```python
from build123d import *

# Parameters (mm, degrees)
SKETCH2_R           = 3.2639
BOSS_EXTRUDE1_DEPTH = 25.0031
SKETCH3_R           = 15.875
CUT_EXTRUDE1_DEPTH  = 13.7
CHAMFER1_SIZE       = 0.5
CHAMFER2_SIZE       = 0.5


with BuildPart() as part:
    # Sketch2 → Boss-Extrude1 (new body)
    with BuildSketch(Plane.XY):
        with BuildLine():
            Line((-6.35, 23.8125), (-6.35, -23.8114))
            ThreePointArc((-6.35, -23.8114), (0, -30.1614), (6.35, -23.8114))
            Line((6.35, -23.8114), (6.35, 23.8125))
            ThreePointArc((6.35, 23.8125), (0, 30.1625), (-6.35, 23.8125))
        make_face()
        with Locations((0, -23.8114)):
            Circle(SKETCH2_R, mode=Mode.SUBTRACT)
        with Locations((0, 23.8125)):
            Circle(SKETCH2_R, mode=Mode.SUBTRACT)
    extrude(amount=BOSS_EXTRUDE1_DEPTH)

    # Sketch3 → Cut-Extrude1 (cut, through all)
    with BuildSketch(Plane(origin=(6.35, 0, 0), x_dir=(0, 0, -1), z_dir=(1, 0, 0))):
        Circle(SKETCH3_R)
    extrude(amount=-CUT_EXTRUDE1_DEPTH, mode=Mode.SUBTRACT)

    # Chamfer1
    chamfer1_edges = [part.edges().sort_by_distance(p)[0] for p in [
        (6.35, 0, 15.875),
    ]]
    chamfer(chamfer1_edges, length=CHAMFER1_SIZE)

    # Chamfer2
    chamfer2_edges = [part.edges().sort_by_distance(p)[0] for p in [
        (-6.35, 0, 15.875),
    ]]
    chamfer(chamfer2_edges, length=CHAMFER2_SIZE)


solid = part.part
```
Design review of the part built by this model. Coordinates are the model's own, in mm. Coordinates: 2 decimals unless noted, no trailing zeros. Loops run counter-clockwise (first coordinate to the right, second up) from the corner with the lowest first, then second, coordinate; pieces in that order, holes last. Notation, with made-up numbers: (62.25, 87) -> (68.25, 87) arc R6 cw to (68.25, 97) -> close; hole circle Ø8 at (51.5, 56.5). An arc over 180 degrees is marked (long way). Answer as a JSON object with one key per item and string values.
Q1. Take a section at D-D on y = -23. Give the boundary of the cut face in (x, z), plus the area to 3 significant figures.
Answer block:
{"outline": "(-6.35, 0) -> (-3.16, 0) -> (-3.16, 25) -> (-6.35, 25) -> close; (3.16, 0) -> (6.35, 0) -> (6.35, 25) -> (3.16, 25) -> close", "area": "159 mm^2"}
Q2. The part is to be moulded in two halves that separate along Y. For faces 1 (the flat face through (-6.35, 0, 18)), 2 (the cylindrical face through (-0.425, -20.575, 12.327)), 3 (the cylindrical face through (-0.14, -30.16, 12.33)), say which applies: +Y half, -Y half, draft (parallel to the pull), parting line (faces both ways), or undercut.
Answer block:
{"face 1": "draft", "face 2": "undercut", "face 3": "-Y half"}
Q3. Take a section at A-A on x = 0. Give the number of separate pieces and of enclosed holes in the cut face, plus the area to 3 significant figures.
Answer block:
{"separate pieces": "3", "enclosed holes": "0", "area": "786 mm^2"}
Q4. To check wall thickness, follow L1, parallel to Y at x = 0, z = 18.5; L2, parallel to Y at x = 0, z = 9; L3, parallel to Y at x = 0.5, z = 6.5. State the ranges of each line that lie inside material, in increasing order.
Answer block:
{"L1": "y = -30.16 to -27.08, -20.55 to 20.55, 27.08 to 30.16", "L2": "y = -30.16 to -27.08, -20.55 to -13.08, 13.08 to 20.55, 27.08 to 30.16", "L3": "y = -30.14 to -27.04, -20.59 to -14.48, 14.48 to 20.59, 27.04 to 30.14"}
Q5. Take a section at C-C on y = 0. Give the boundary of the cut face in (x, z) (3 decimals), plus the area to 3 significant figures.
Answer block:
{"outline": "(-6.35, 16.375) -> (-5.85, 15.875) -> (5.85, 15.875) -> (6.35, 16.375) -> (6.35, 25.003) -> (-6.35, 25.003) -> close", "area": "116 mm^2"}
Q6. Clearance check with flat-ended pins moving along their axes: pin 1 Ø2 at (x, z) = (1.5, 7) entering from -Y; pin 2 Ø2 at (x, y) = (2, 12.5) entering from -Z; pin 3 Ø5 at (x, z) = (5, 9.5) entering from -Y; pin 4 Ø4 at (x, y) = (0, 23.81) entering from +Z. State where each tip first meets the part, or that it passes through.
Answer block:
{"pin 1": "stops at y = -30.14", "pin 2": "stops at z = 8.35", "pin 3": "stops at y = -29.65", "pin 4": "passes through"}
Q7. Take a section at B-B on z = 17.5. Give the boundary of the cut face in (x, y), plus the area to 3 significant figures.
Answer block:
{"outline": "(-6.35, -23.81) arc R6.35 ccw to (6.35, -23.81) -> (6.35, 23.81) arc R6.35 ccw to (-6.35, 23.81) -> close; hole circle Ø6.53 at (0, -23.81); hole circle Ø6.53 at (0, 23.81)", "area": "665 mm^2"}
